from build123d import *

# Parameters (mm, degrees)
BOSS_EXTRUDE8_DEPTH = 6
SKETCH7_R           = 5
CUT_EXTRUDE3_DEPTH  = 14
SKETCH8_R           = 1.5
CUT_EXTRUDE4_DEPTH  = 97.076913025
CHAMFER3_SIZE       = 5
FILLET4_R           = 2


with BuildPart() as part:
    # Sketch1 → Boss-Extrude8 (new, symmetric)
    with BuildSketch(Plane.XY):
        Polygon((10, -8), (88.038475773, -30), (80, 0), (88.038475773, 30), (10, 8), (0, 8), (0, -8), align=None)
    extrude(amount=BOSS_EXTRUDE8_DEPTH, both=True)

    # Sketch7 → Cut-Extrude3 (cut)
    with BuildSketch(Plane.ZY):
        Circle(SKETCH7_R)
    extrude(amount=-CUT_EXTRUDE3_DEPTH, mode=Mode.SUBTRACT)

    # Sketch8 → Cut-Extrude4 (cut, through all)
    with BuildSketch(Plane(origin=(0, 8, 0), x_dir=(1, 0, 0), z_dir=(0, 1, 0))):
        with Locations(Location((6, 0, 0), (0, 0, 180))):
            Circle(SKETCH8_R)
    extrude(amount=-CUT_EXTRUDE4_DEPTH, mode=Mode.SUBTRACT)

    # Chamfer3
    chamfer3_edges = [part.edges().sort_by_distance(p)[0] for p in [
        (49.019237886, -19, 6),
        (84.019237886, -15, 6),
        (84.019237886, 15, 6),
        (49.019237886, 19, 6),
        (49.019237886, 19, -6),
        (84.019237886, 15, -6),
        (84.019237886, -15, -6),
        (49.019237886, -19, -6),
    ]]
    chamfer(chamfer3_edges, length=CHAMFER3_SIZE)

    # Fillet4
    fillet4_edges = [part.edges().sort_by_distance(p)[0] for p in [
        (14.213662503, -8, 6),
        (14.213662503, 8, 6),
        (14.213662503, -8, -6),
        (14.213662503, 8, -6),
    ]]
    fillet(fillet4_edges, radius=FILLET4_R)


solid = part.part
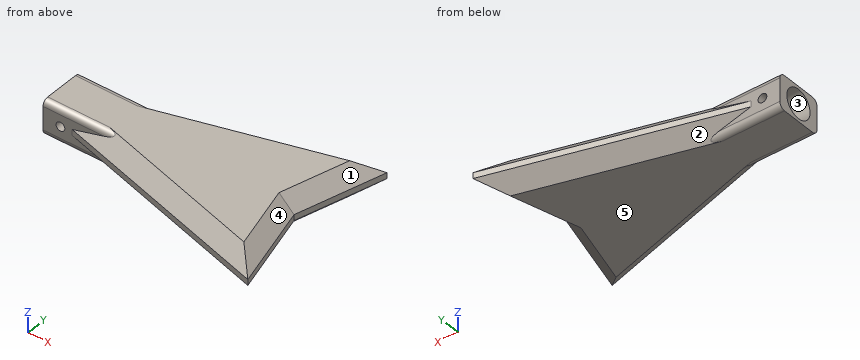
Design review of the part built by this model. Coordinates are the model's own, in mm. Face numbers are marked on the shaded views. A direction names the side the tool comes from. Give positions to 0.01 mm unless a question says otherwise; leave off trailing zeros. Loops run counter-clockwise (first coordinate to the right, second up) from the corner with the lowest first, then second, coordinate; pieces in that order, holes last. Notation, with made-up numbers: (55, -2) - (70, -2) arc R21 ccw to (70, 27) - close; hole circle Ø7 at (19, 76). An arc over 180 degrees is marked (long way). Use CSV: the item, a comma, the result in double quotes. Start each with the question number.
1. Insertion check: P1, Ø1, axis at x = 40, z = 3.5, coming from the -Y side; P2, Ø8, axis at x = 28, y = 8, coming from the -Z side; P3, Ø2, axis at x = 58.5, z = 1, coming from the -Y side; P4, Ø2, axis at y = 23.5, z = -2.5, coming from the +X side. Each pin has a flat end and moves straight along its axis. Give the tip position at first contact, or say it passes through.
2. Add section C-C (y = 7). State the section outline as (x, z) points, plus the area to 3 significant figures.
3. Add section D-D (x = 52). State the section outline as (y, z) points, plus the area to 3 significant figures.
4. Add section A-A (z = 0). State the section outline as (x, y) points, plus the area to 3 significant figures.
5. Draft analysis for pull direction Z (two halves, no side actions). For the marked faces 1, 2 and 3, state which applies: released by +Z, released by -Z, zero draft, split by the parting line, or undercut.
6. Machinability: for the marked faces 4 and 5, which of the approach directions +Z, -Z, +X, -X, +Y, -Y give a long, thin tool a straight path to every point of the face, cutting with its end or side? Answer none if there is none.
7. Wall thickness on L1, parallel to Z at x = 6, y = 6.15; L2, parallel to X at y = -6.55, z = 0; L3, parallel to Y at x = 5, z = -2.5: over which ranges is each line inside the solid? List them lowest first.
8. Add section B-B (x = 6). State the section outline as (y, z) points.
Results found:
1,P1,"stops at y = -14.4"
1,P2,"stops at z = -6"
1,P3,"stops at y = -21.95"
1,P4,"stops at x = 85.81"
2,outline,"(0, -5.73) - (23.89, -5.73) - (24.88, -6) - (76.7, -6) - (81.88, -1) - (81.88, 1) - (76.7, 6) - (24.88, 6) - (23.89, 5.73) - (0, 5.73) - close; hole circle Ø3 at (6, 0)"
2,area,"936 mm²"
3,outline,"(-19.84, -1) - (-14.65, -6) - (14.65, -6) - (19.84, -1) - (19.84, 1) - (14.65, 6) - (-14.65, 6) - (-19.84, 1) - close"
3,area,"424 mm²"
4,outline,"(0, -8) - (4.5, -8) - (4.5, -5) - (0, -5) - close; (0, 5) - (4.5, 5) - (4.5, 8) - (0, 8) - close; (7.5, -8) - (10, -8) - (88.04, -30) - (80, 0) - (88.04, 30) - (10, 8) - (7.5, 8) - (7.5, 5) - (14, 5) - (14, -5) - (7.5, -5) - close"
4,area,"2,730 mm²"
5,face 1,"released by +Z"
5,face 2,"released by -Z"
5,face 3,"undercut"
6,face 4,"+Z, +X"
6,face 5,"-Z, +X, -X, +Y, -Y"
7,L1,"z = -5.99 to -1.5, 1.5 to 5.99"
7,L2,"x = 0 to 4.5, 7.5 to 81.76"
7,L3,"y = -8 to -4.33, 4.33 to 8"
8,outline,"(-8, -4) arc R2 ccw to (-6, -6) - (6, -6) arc R2 ccw to (8, -4) - (8, -1.5) - (4.77, -1.5) arc R5 cw to (-4.77, -1.5) - (-8, -1.5) - close; (-8, 1.5) - (-4.77, 1.5) arc R5 cw to (4.77, 1.5) - (8, 1.5) - (8, 4) arc R2 ccw to (6, 6) - (-6, 6) arc R2 ccw to (-8, 4) - close"
